Part model, mm, in its own coordinate system. Coordinates: 2 decimals unless noted, no trailing zeros. Order: outer loops, then holes, each group sorted by start corner. A loop starts at its lowest first (then second) coordinate and runs counter-clockwise, first axis right, second up.
Autodesk Inventor part; units mm, degrees
ref_plane "YZ Plane" through (0, 0, 0) normal (1, 0, 0) x (0, 1, 0)
ref_plane "XZ Plane" through (0, 0, 0) normal (0, 1, 0) x (-1, 0, 0)
ref_plane "XY Plane" through (0, 0, 0) normal (0, 0, 1) x (1, 0, 0)
sketch "main" plane through (0, 0, 0) normal (0, 0, 1) x (1, 0, 0)
  circle A0 centre (-13.3607, 90.7974) radius 2.1844
  circle A1 centre (-19.7107, 109.8474) radius 2.1844
  circle A2 centre (-19.7107, 122.5474) radius 2.1358
  circle A3 centre (-19.7107, 147.9474) radius 2.1844
  circle A4 centre (-19.7107, 135.2474) radius 2.1844
  circle A5 centre (-19.7107, 173.3474) radius 2.1844
  circle A6 centre (-19.7107, 160.6474) radius 2.1844
  circle A7 centre (-13.3607, 65.3974) radius 2.1844
  circle A8 centre (-19.7107, 46.3474) radius 2.1844
  circle A9 centre (-19.7107, 33.6474) radius 2.1844
  circle A10 centre (-19.7107, 20.9474) radius 2.1844 construction
  line L0 (-1.5114, 189.2224) -> (37.374, -79.744)
  line L1 (-40.3482, -167.9651) -> (-40.3482, 159.8585)
  circle A11 centre (-13.3607, 1.8974) radius 2.1844 construction
  circle A12 centre (-13.3607, -23.5026) radius 2.1844 construction
  circle A13 centre (-19.7107, -42.5526) radius 2.1844 construction
  circle A14 centre (-19.7107, -67.9526) radius 2.1844 construction
  circle A15 centre (31.0893, -80.6526) radius 2.1844
  circle A16 centre (-19.7107, -55.2526) radius 2.1844 construction
  circle A17 centre (-13.3607, -87.0026) radius 2.1844 construction
  circle A18 centre (-13.3607, -112.4026) radius 2.1844 construction
  circle A19 centre (-19.7107, -131.4526) radius 2.1844 construction
  circle A20 centre (-19.7107, -144.1526) radius 2.1844 construction
  line L2 (37.374, -79.744) -> (37.4393, -144.1462)
  arc A21 (35.5805, -148.6417) -> (37.4393, -144.1462) centre (31.0893, -144.1526) ccw
  arc A22 (37.3758, -81.5485) -> (37.374, -79.744) centre (31.0893, -80.6526) ccw
  circle A23 centre (-19.7107, -156.8526) radius 2.1844 construction
  arc A24 (-40.3482, -167.9651) -> (-38.4883, -172.4553) centre (-33.9982, -167.9651) ccw
  line L3 (35.5805, -148.6417) -> (-2.5106, -186.7506)
  line L4 (-2.5106, -186.7506) -> (-1.346, -186.7506) construction
  arc A25 (-7.3374, -188.6026) -> (-2.5106, -186.7506) centre (-7.0018, -182.2615) ccw
  line L5 (-24.1929, -186.7506) -> (-38.4883, -172.4553)
  line L6 (-7.3374, -188.6026) -> (-19.7047, -188.6066)
  arc A26 (-24.2008, -186.7428) -> (-19.7047, -188.6066) centre (-19.7067, -182.2566) ccw
  circle A27 centre (31.0893, -144.1526) radius 2.1844
  arc A28 (-19.7107, 192.3974) -> (-25.3223, 189.0193) centre (-19.7107, 186.0474) ccw
  arc A29 (-0.8373, 184.5599) -> (-7.0107, 192.3974) centre (-7.0107, 186.0474) ccw
  arc A30 (-39.979, 161.3445) -> (-40.3482, 159.8585) centre (-37.1732, 159.8585) ccw
  line L7 (-39.979, 161.3445) -> (-25.3223, 189.0193)
  line L8 (-19.7107, 192.3974) -> (-7.0107, 192.3974)
  circle A31 centre (-19.7107, 173.3474) radius 4.2164
  circle A32 centre (-19.7107, 160.6474) radius 4.2166
  circle A33 centre (-19.7107, 147.9474) radius 4.2167
  circle A34 centre (-19.7107, 135.2474) radius 4.2169
  circle A35 centre (-19.7107, 122.5474) radius 4.217
  circle A36 centre (-19.7107, 109.8474) radius 4.2171
  circle A37 centre (-13.3607, 90.7974) radius 4.2164
  circle A38 centre (-13.3607, 65.3974) radius 4.2167
  circle A39 centre (-19.7107, 46.3474) radius 4.2178
  circle A40 centre (-19.7107, 33.6474) radius 4.2179
  circle A41 centre (-19.7107, 20.9474) radius 4.2181
  circle A42 centre (-13.3607, 1.8974) radius 4.2173
  circle A43 centre (-13.3607, -23.5026) radius 4.2176
  circle A44 centre (-19.7107, -42.5526) radius 4.2188
  circle A45 centre (-19.7107, -55.2526) radius 4.2189
  circle A46 centre (-19.7107, -67.9526) radius 4.219
  circle A47 centre (-13.3607, -87.0026) radius 4.2183
  circle A48 centre (-13.3607, -112.4026) radius 4.2186
  circle A49 centre (-19.7107, -131.4526) radius 4.2197
  circle A50 centre (-19.7107, -144.1526) radius 4.2198
  circle A51 centre (-19.7107, -156.8526) radius 4.22
  point P0 (-9.7209, -19.0127)
  dimension "d0" = 135
  dimension "d1" = 135
  dimension "d2" = 6.35
  dimension "d3" = 3.175
  dimension "d4" = 8.4328
  dimension "d5" = 8.4328
sketch "Sketch1" plane through (0, 0, 0) normal (0, 0, 1) x (1, 0, 0)
  circle A0 centre (95.2501, 6.349) radius 2.1844
  circle A1 centre (76.2, -0.0008) radius 2.1844
  circle A2 centre (63.5, -0.0007) radius 2.1358
  circle A3 centre (38.1, -0.0004) radius 2.1844
  circle A4 centre (50.8, -0.0005) radius 2.1844
  circle A5 centre (12.7, -0.0001) radius 2.1844
  circle A6 centre (25.4, -0.0003) radius 2.1844
  circle A7 centre (120.6501, 6.3487) radius 2.1844
  circle A8 centre (139.7, -0.0015) radius 2.1844
  circle A9 centre (152.4, -0.0016) radius 2.1844
  circle A10 centre (165.1, -0.0018) radius 2.1844 construction
  line L0 (-3.1748, 18.1993) -> (265.792, 57.0818)
  line L1 (354.0123, -20.6413) -> (26.1886, -20.6378)
  circle A11 centre (184.1501, 6.348) radius 2.1844 construction
  circle A12 centre (209.5501, 6.3478) radius 2.1844 construction
  circle A13 centre (228.6, -0.0024) radius 2.1844 construction
  circle A14 centre (254, -0.0027) radius 2.1844 construction
  circle A15 centre (266.7005, 50.7972) radius 2.1844
  circle A16 centre (241.3, -0.0026) radius 2.1844 construction
  circle A17 centre (273.0501, 6.3471) radius 2.1844 construction
  circle A18 centre (298.4501, 6.3468) radius 2.1844 construction
  circle A19 centre (317.5, -0.0034) radius 2.1844 construction
  circle A20 centre (330.2, -0.0035) radius 2.1844 construction
  line L2 (265.792, 57.0818) -> (330.1942, 57.1465)
  arc A21 (334.6897, 55.2876) -> (330.1942, 57.1465) centre (330.2005, 50.7965) ccw
  arc A22 (267.5964, 57.0836) -> (265.792, 57.0818) centre (266.7005, 50.7972) ccw
  circle A23 centre (342.9, -0.0036) radius 2.1844 construction
  arc A24 (354.0123, -20.6413) -> (358.5024, -18.7814) centre (354.0123, -14.2913) ccw
  line L3 (334.6897, 55.2876) -> (372.7981, 17.1961)
  line L4 (372.7981, 17.1961) -> (372.7982, 18.3607) construction
  arc A25 (374.6501, 12.3693) -> (372.7981, 17.1961) centre (368.309, 12.705) ccw
  line L5 (372.7979, -4.4862) -> (358.5024, -18.7814)
  line L6 (374.6501, 12.3693) -> (374.6539, 0.0019)
  arc A26 (372.7901, -4.4941) -> (374.6539, 0.0019) centre (368.3039, 0) ccw
  circle A27 centre (330.2005, 50.7965) radius 2.1844
  arc A28 (-6.35, 0.0001) -> (-2.972, -5.6116) centre (0, 0) ccw
  arc A29 (1.4877, 18.8733) -> (-6.3499, 12.7001) centre (0.0001, 12.7) ccw
  arc A30 (24.7027, -20.2686) -> (26.1886, -20.6378) centre (26.1887, -17.4628) ccw
  line L7 (24.7027, -20.2686) -> (-2.972, -5.6116)
  line L8 (-6.35, 0.0001) -> (-6.3499, 12.7001)
  circle A31 centre (12.7, -0.0001) radius 4.2164
  circle A32 centre (25.4, -0.0003) radius 4.2166
  circle A33 centre (38.1, -0.0004) radius 4.2167
  circle A34 centre (50.8, -0.0005) radius 4.2169
  circle A35 centre (63.5, -0.0007) radius 4.217
  circle A36 centre (76.2, -0.0008) radius 4.2171
  circle A37 centre (95.2501, 6.349) radius 4.2164
  circle A38 centre (120.6501, 6.3487) radius 4.2167
  circle A39 centre (139.7, -0.0015) radius 4.2178
  circle A40 centre (152.4, -0.0016) radius 4.2179
  circle A41 centre (165.1, -0.0018) radius 4.2181
  circle A42 centre (184.1501, 6.348) radius 4.2173
  circle A43 centre (209.5501, 6.3478) radius 4.2176
  circle A44 centre (228.6, -0.0024) radius 4.2188
  circle A45 centre (241.3, -0.0026) radius 4.2189
  circle A46 centre (254, -0.0027) radius 4.219
  circle A47 centre (273.0501, 6.3471) radius 4.2183
  circle A48 centre (298.4501, 6.3468) radius 4.2186
  circle A49 centre (317.5, -0.0034) radius 4.2197
  circle A50 centre (330.2, -0.0035) radius 4.2198
  circle A51 centre (342.9, -0.0036) radius 4.22
  point P0 (0, 0)
extrude "Extrusion1" add sketch "Sketch1" along normal blind 1.5875 contours L0 L2 A21 L3 A25 L6 A26 L5 A24 L1 A30 L7 A28 L8 A29
properties part number "skirt" material "Acetal Resin, White"
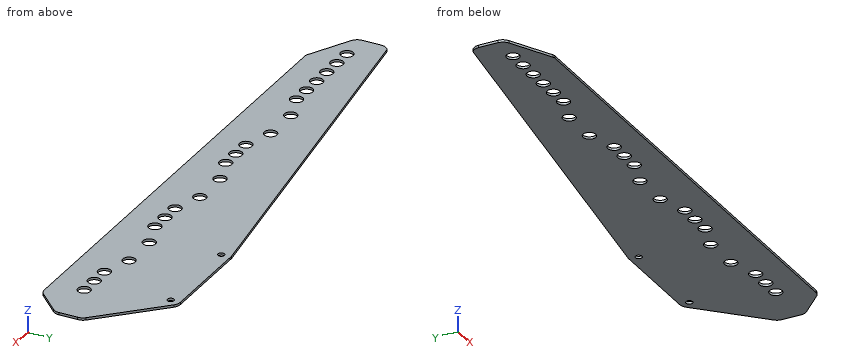
Q1. Wall check: line 1 along Y through (x, z) = (330, 1); line 2 along Y through (x, z) = (298, 0.4); line 3 along Y through (x, z) = (99, 0.8). Give the ranges that are in metal, low to high.
Results list:
line 1: y = -20.64 to -4.22, 4.21 to 48.62, 52.97 to 57.15
line 2: y = -20.64 to 2.15, 10.54 to 57.11
line 3: y = -20.64 to 4.42, 8.28 to 32.97
Q2. Cut at D-D on z = 0.55. Count the separate pieces of the cut face and the enclosed holes in it, and give its area (3 significant figures).
Results list:
separate pieces: 1
enclosed holes: 23
area: 21,700 mm2
Q3. Cut at C-C on y = -14.5. Write the cut outline in (x, z), and give its area (3 significant figures).
Results list:
outline: (13.81, 0) - (362.78, 0) - (362.78, 1.59) - (13.81, 1.59) - close
area: 554 mm2
Q4. Pin check, flat tip, straight feed: pin 1 Ø7.5 at (x, y) = (184.15, 6.35) entering from -Z. Stop position of the tip, or through.
Results list:
pin 1: passes through
Q5. Cut at B-B on x = 139.7. Write the cut outline in (y, z).
Results list:
outline: (-20.64, 0) - (-4.22, 0) - (-4.22, 1.59) - (-20.64, 1.59) - close; (4.22, 0) - (38.85, 0) - (38.85, 1.59) - (4.22, 1.59) - close
Q6. Cut at A-A on x = 317.5. Write the cut outline in (y, z), and give its area (3 significant figures).
Results list:
outline: (-20.64, 0) - (-4.22, 0) - (-4.22, 1.59) - (-20.64, 1.59) - close; (4.22, 0) - (57.13, 0) - (57.13, 1.59) - (4.22, 1.59) - close
area: 110 mm2
